from build123d import *

# Parameters (mm, degrees)
F0_R            = 127
F1_DEPTH        = 25.4
F2_R            = 101.6
F3_DEPTH        = 25.401
F5_DEPTH        = 19.05
F5_COPIES_COUNT = 20


# Not quite as in the source:
# - a pattern or mirror of a feature is missing from the dataset's text; its kind, count and spacing are read off the source's solid


with BuildPart() as f1:
    # F0 (on Front) → F1 (new body)
    with BuildSketch(Plane.XZ):
        Circle(F0_R)
    extrude(amount=F1_DEPTH)

    # F2 (on face) → F3 (cut, through all)
    with BuildSketch(Plane.XZ.offset(25.4)):
        Circle(F2_R)
    extrude(amount=-F3_DEPTH, mode=Mode.SUBTRACT)

    # F4 (on face) → F5 (cut)
    with BuildSketch(Plane.XZ.offset(25.4)):
        with BuildLine():
            ThreePointArc((-8.1511862482, 114.5919902466), (0, 106.7252035251), (8.1511862482, 114.5919902466))
            ThreePointArc((8.1511862482, 114.5919902466), (0, 114.8815305693), (-8.1511862482, 114.5919902466))
        make_face()
        with BuildLine():
            ThreePointArc((-8.1511862482, 114.5919902466), (0, 114.8815305693), (8.1511862482, 114.5919902466))
            ThreePointArc((8.1511862482, 114.5919902466), (8.1550417439, 114.736737591), (8.1563270441, 114.8815305693))
            ThreePointArc((8.1563270441, 114.8815305693), (-0.1447929783, 123.0365723132), (-8.1511862482, 114.5919902466))
        make_face()
    f5 = extrude(amount=-F5_DEPTH, mode=Mode.SUBTRACT)

    # F5_copies: F5 ×20 about axis
    f5_copies_axis = Axis((0, 0, 0), (0, 1, 0))
    for i in range(1, F5_COPIES_COUNT):
        add(f5.rotate(f5_copies_axis, i * 360 / F5_COPIES_COUNT), mode=Mode.SUBTRACT)


solid = f1.part
Work out the finished part from the listing and answer in its coordinate system (mm). A direction names the side the tool comes from. Round coordinates to 2 decimals unless told otherwise and drop trailing zeros. Order: outer loops, then holes, each group sorted by start corner. A loop starts at its lowest first (then second) coordinate and runs counter-clockwise, first axis right, second up. Notation, with made-up numbers: M 79,15 L 138,15 A19 ccw 138,52 Z; hole C 48.5,17.5 d4. An arc over 180 degrees is marked long. Put each result on its own line as item: value. Start each with the question number.
Q1. Straight lines are drawn through the part: L1, parallel to Z at x = 0, y = -18.5; L2, parallel to X at y = -16.75, z = 39; L3, parallel to X at y = -19.5, z = -93.5. For each, find the intervals that lie inside material, in ascending order. Write a range as [from, to].
Q2. Section A-A, the plane z = 0 is taken. Write down the section's boundary in (x, y).
Q3. For a pull along Z with two mould halves and no side action, classify faces 3 (the flat face through (37, -25.4, 95)), 4 (the flat face through (36, -6.35, -109)), 5 (the cylindrical face through (-27.53, -12.52, -123.98)), 6 (the flat face through (115, -6.35, 0)) as pulls with the +Z half, pulls with the -Z half, needs draft (parallel to the pull), parting line crosses it, or undercut.
Q4. Flat-ended cylindrical pins translate along their axes: pin 1 (5 mm diameter, centred on x = 34, z = 113, fed in from -Y); pin 2 (10 mm diameter, centred on y = -17, z = -101, fed in from +X); pin 3 (1.5 mm diameter, centred on y = -12, z = -79, fed in from +X). Find the tip coordinate at first contact, or state that the pin passes through.
Q5. Section C-C, the plane y = -18.75 is taken. Give the number of separate pieces and of enclosed holes in the cut face, and give its area (3 significant figures).
Q6. Section B-B, the plane x = 0 is taken. Write down the section's boundary in (y, z).
Q7. A tool of negligible diameter and unlimited length cuts with its end or side. For faces 1 (the flat face through (-93, -6.35, -68)), 2 (the cylindrical face through (-22.025, -12.878, -99.184)), from which of +Z, -Z, +X, -X, +Y, -Y can it reach the whole face along a straight path? Write none if from no direction.
Findings below:
1. L1: z = [-127, -123.04], [-106.73, -101.6], [101.6, 106.73], [123.04, 127]
1. L2: x = [-120.86, -116.63], [-101.89, -93.82], [93.82, 101.89], [116.63, 120.86]
1. L3: x = [-85.95, -75.66], [-59.39, -39.75], [39.75, 59.39], [75.66, 85.95]
2. outline: M -127,-25.4 L -123.04,-25.4 L -123.04,-6.35 L -106.73,-6.35 L -106.73,-25.4 L -101.6,-25.4 L -101.6,0 L -127,0 Z; M 101.6,-25.4 L 106.73,-25.4 L 106.73,-6.35 L 123.04,-6.35 L 123.04,-25.4 L 127,-25.4 L 127,0 L 101.6,0 Z
3. face 3: needs draft
3. face 4: undercut
3. face 5: parting line crosses it
3. face 6: undercut
4. pin 1: stops at y = -6.35
4. pin 2: stops at x = 83.14
4. pin 3: stops at x = 100.03
5. separate pieces: 1
5. enclosed holes: 21
5. area: 14,100 mm^2
6. outline: M -25.4,-127 L 0,-127 L 0,-101.6 L -25.4,-101.6 L -25.4,-106.73 L -6.35,-106.73 L -6.35,-123.04 L -25.4,-123.04 Z; M -25.4,101.6 L 0,101.6 L 0,127 L -25.4,127 L -25.4,123.04 L -6.35,123.04 L -6.35,106.73 L -25.4,106.73 Z
7. face 1: -Y
7. face 2: +Y, -Y
